from build123d import *

# Parameters (mm, degrees)
BASE_DEPTH                 = 20
CHAMFER1_SIZE              = 1
F_3_2_3_2_MOUNTSIDE_D      = 3.2
F_3_2_3_2_CABLECHAINSIDE_D = 3.2


with BuildPart() as part:
    # Sketch1 → Base (new body)
    with BuildSketch(Plane.XY):
        Polygon((0, 0), (35, 0), (35, 2), (2, 2), (2, 15), (0, 15), align=None)
    extrude(amount=BASE_DEPTH)

    # Chamfer1
    chamfer1_edges = [part.edges().sort_by_distance(p)[0] for p in [
        (35, 1, 20),
        (1, 15, 20),
        (1, 15, 0),
        (35, 1, 0),
    ]]
    chamfer(chamfer1_edges, length=CHAMFER1_SIZE)

    # Ø3.2 (3.2) MountSide (through all)
    with Locations(Plane.ZY):
        with Locations((5.75, 11), (14.25, 11)):
            Hole(F_3_2_3_2_MOUNTSIDE_D / 2)

    # Ø3.2 (3.2) CableChainSide (through all)
    with Locations(Plane(origin=(0, 0, 0), x_dir=(-1, 0, 0), z_dir=(0, -1, 0))):
        with Locations((-28.75, -9.3), (-21.25, -16)):
            Hole(F_3_2_3_2_CABLECHAINSIDE_D / 2)


solid = part.part
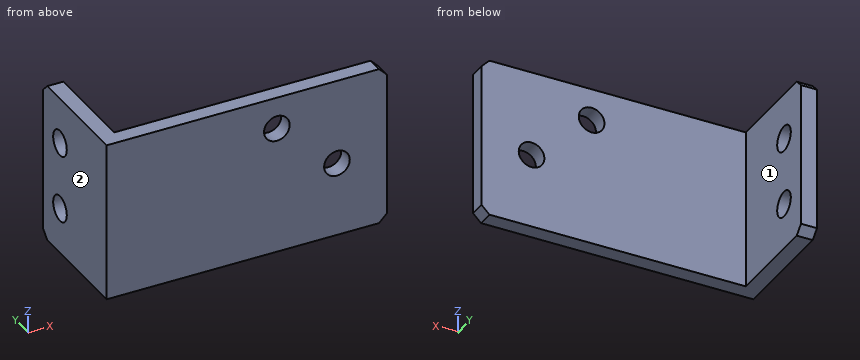
The listing builds one solid part. Answer for the finished solid, in the listing's coordinates (mm). Face numbers are marked on the shaded views. A direction names the side the tool comes from. Give positions to 0.01 mm unless a question says otherwise; leave off trailing zeros. Write each loop counter-clockwise with the first axis right and the second up, starting at its lowest first coordinate (ties: lowest second). Pieces come first, ordered by that corner, then holes.
1) Section B-B (y = 1) is taken. Write down the section's boundary in (x, z), and give its area (3 significant figures).
2) A tool of negligible diameter and unlimited length cuts with its end or side. For the marked faces 1 and 2, from which of +Z, -Z, +X, -X, +Y, -Y can it reach the whole face along a straight path? Write none if from no direction.
3) Section C-C (x = 28.75) is taken. Write down the section's boundary in (y, z), and give its area (3 significant figures).
4) Find the intervals of material crossed by L1, parallel to Z at x = 28.75, y = 1.1; L2, parallel to Z at x = 21.25, y = 0.7; L3, parallel to Y at x = 1, z = 5.75, in increasing order.
5) Section D-D (y = 11) is taken. Write down the section's boundary in (x, z), and give its area (3 significant figures).
6) Section A-A (z = 9.3) is taken. Write down the section's boundary in (x, y).
7) Given P1, Ø3, axis at x = 28.75, z = 9.3, coming from the +Y side; P2, Ø1, axis at y = 3, z = 5.5, coming from the +X side; P3, Ø3, axis at x = 30.5, z = 17, coming from the +Y side, each flat-ended and moving along its own axis, determine where each tip first touches the part or whether it passes through.
Response:
1. outline: (0, 0) - (34, 0) - (35, 1) - (35, 19) - (34, 20) - (0, 20) - close; hole circle Ø3.2 at (21.25, 16); hole circle Ø3.2 at (28.75, 9.3)
1. area: 683 mm2
2. face 1: +Z, -Z, +X, +Y
2. face 2: +Z, -Z, -X, +Y, -Y
3. outline: (0, 0) - (2, 0) - (2, 7.7) - (0, 7.7) - close; (0, 10.9) - (2, 10.9) - (2, 20) - (0, 20) - close
3. area: 33.6 mm2
4. L1: z = 0 to 7.7, 10.9 to 20
4. L2: z = 0 to 14.4, 17.6 to 20
4. L3: y = 0 to 9.4, 12.6 to 15
5. outline: (0, 0) - (2, 0) - (2, 4.15) - (0, 4.15) - close; (0, 7.35) - (2, 7.35) - (2, 12.65) - (0, 12.65) - close; (0, 15.85) - (2, 15.85) - (2, 20) - (0, 20) - close
5. area: 27.2 mm2
6. outline: (0, 0) - (27.15, 0) - (27.15, 2) - (2, 2) - (2, 15) - (0, 15) - close; (30.35, 0) - (35, 0) - (35, 2) - (30.35, 2) - close
7. P1: passes through
7. P2: stops at x = 2
7. P3: stops at y = 2
